The figure shows three views and two pictorial views of one solid part (mm, origin at its lowest corner). Answer the questions. A direction names the side the tool comes from. Coordinates: 2 decimals unless noted, no trailing zeros. Write each loop counter-clockwise with the first axis right and the second up, starting at its lowest first coordinate (ties: lowest second). Pieces come first, ordered by that corner, then holes. Notation, with made-up numbers: (-19.75, 56.25) - (30.25, 56.25) arc R34 cw to (30.25, 93.25) - close; hole circle Ø7 at (-27.5, 15). An arc over 180 degrees is marked (long way). Use a Markdown table: item, result. Add a question column.
(1) The part is cut by section C-C, the plane z = 17.75. Give the vertices of the cut face in (x, y), then the cut area to 3 significant figures.
(2) Given pin 1 Ø5 at (y, z) = (50.5, 8) entering from +X; pin 2 Ø2 at (x, z) = (74.5, 14) entering from -Y; pin 3 Ø8 at (y, z) = (36.5, 15.5) entering from -X, each flat-ended and moving along its own axis, determine where each tip first touches the part or whether it passes through.
(3) The part is cut by section D-D, the plane y = 88. Give the vertices of the cut face in (x, z), then the cut area to 3 significant figures.
(4) The part is cut by section B-B, the plane x = 48. Give the vertices of the cut face in (y, z).
(5) A tool of negligible diameter and unlimited length cuts with its end or side. For the marked faces 1, 2 and 3, from which of +Z, -Z, +X, -X, +Y, -Y can it reach the whole face along a straight path? Write none if from no direction.
(6) The part is cut by section A-A, the plane y = 48. Give the vertices of the cut face in (x, z).
(7) Find the intervals of material crossed by line 1 (Z direction, x = 39, y = 7.5); line 2 (X direction, y = 47.5, z = 12); line 3 (X direction, y = 88, z = 20.5), in increasing order. Write a range as from..to.
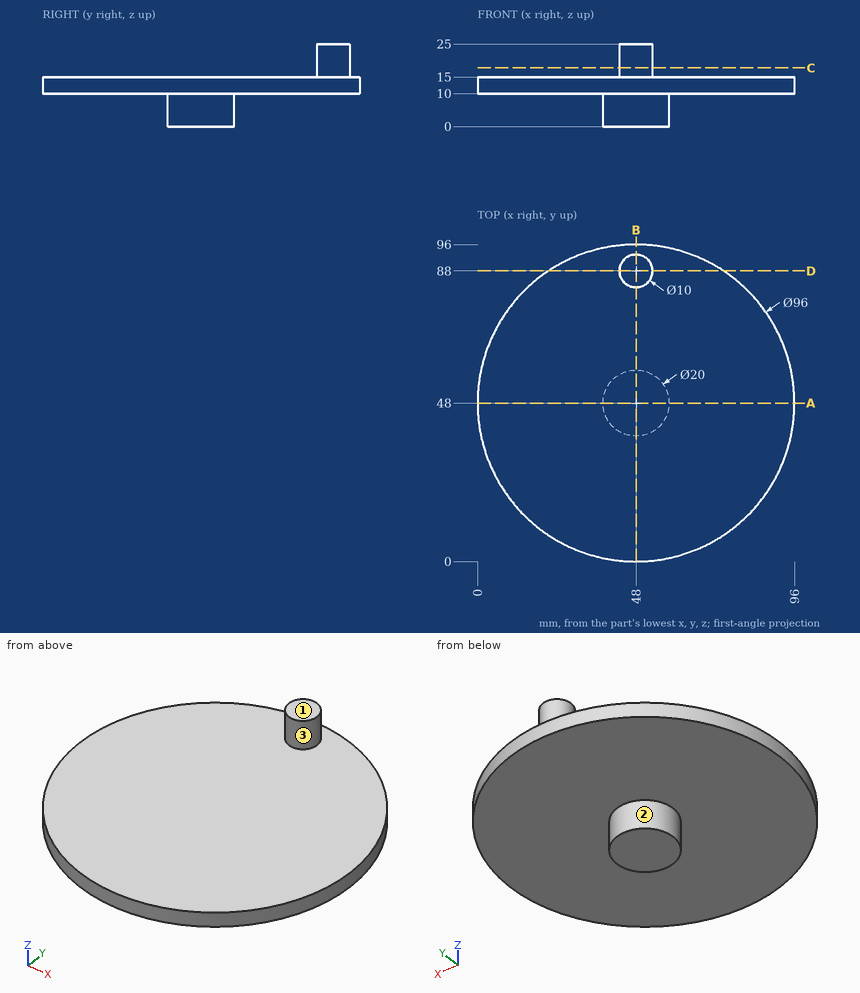
Model answer:
| question | item | result |
|---|---|---|
| 1 | outline | circle Ø10 at (48, 88) |
| 1 | area | 78.5 mm^2 |
| 2 | pin 1 | x = 95.99 |
| 2 | pin 2 | y = 7.33 |
| 2 | pin 3 | x = 0.59 |
| 3 | outline | (21.47, 10) - (74.53, 10) - (74.53, 15) - (53, 15) - (53, 25) - (43, 25) - (43, 15) - (21.47, 15) - close |
| 3 | area | 365 mm^2 |
| 4 | outline | (0, 10) - (38, 10) - (38, 0) - (58, 0) - (58, 10) - (96, 10) - (96, 15) - (93, 15) - (93, 25) - (83, 25) - (83, 15) - (0, 15) - close |
| 5 | face 1 | +Z, +X, -X, +Y, -Y |
| 5 | face 2 | -Z |
| 5 | face 3 | +Z |
| 6 | outline | (0, 10) - (38, 10) - (38, 0) - (58, 0) - (58, 10) - (96, 10) - (96, 15) - (0, 15) - close |
| 7 | line 1 | 10..15 |
| 7 | line 2 | 0..96 |
| 7 | line 3 | 43..53 |
